```python
from build123d import *

# Parameters (mm, degrees)
SKETCH1_W           = 76.2
SKETCH1_H           = 76.2
BOSS_EXTRUDE1_DEPTH = 3.175
SKETCH2_W           = 50.8
SKETCH2_H           = 50.8
CUT_EXTRUDE1_DEPTH  = 6.35
SKETCH3_R           = 2.159
CUT_EXTRUDE2_DEPTH  = 6.35
SKETCH5_R           = 2.159
CUT_EXTRUDE3_DEPTH  = 6.35
SKETCH6_R           = 2.159
CUT_EXTRUDE4_DEPTH  = 54.975


with BuildPart() as part:
    # Sketch1 → Boss-Extrude1 (new body)
    with BuildSketch(Plane.XY):
        Rectangle(SKETCH1_W, SKETCH1_H)
    extrude(amount=BOSS_EXTRUDE1_DEPTH)

    # Sketch2 → Cut-Extrude1 (cut)
    with BuildSketch(Plane(origin=(0, 0, 0), x_dir=(-1, 0, 0), z_dir=(0, 0, -1))):
        with Locations((12.7, 12.7)):
            Rectangle(SKETCH2_W, SKETCH2_H)
    extrude(amount=-CUT_EXTRUDE1_DEPTH, mode=Mode.SUBTRACT)

    # Sketch3 → Cut-Extrude2 (cut)
    with BuildSketch(Plane(origin=(0, 0, 0), x_dir=(-1, 0, 0), z_dir=(0, 0, -1))):
        with Locations((-25.4, -25.4)):
            Circle(SKETCH3_R)
    extrude(amount=-CUT_EXTRUDE2_DEPTH, mode=Mode.SUBTRACT)

    # Sketch5 → Cut-Extrude3 (cut)
    with BuildSketch(Plane(origin=(0, 0, 0), x_dir=(-1, 0, 0), z_dir=(0, 0, -1))):
        with Locations((24.892, -25.4)):
            Circle(SKETCH5_R)
    extrude(amount=-CUT_EXTRUDE3_DEPTH, mode=Mode.SUBTRACT)

    # Sketch6 → Cut-Extrude4 (cut, through all)
    with BuildSketch(Plane.XY.offset(3.175)):
        with Locations((25.4, 0.508)):
            Circle(SKETCH6_R)
        with Locations((25.4, 24.892)):
            Circle(SKETCH6_R)
    extrude(amount=-CUT_EXTRUDE4_DEPTH, mode=Mode.SUBTRACT)


solid = part.part
```
Geometry: final body of the model. Coordinates: model frame, mm. A direction names the side the tool comes from. Give positions to 0.01 mm unless a question says otherwise; leave off trailing zeros. Loops run counter-clockwise (first coordinate to the right, second up) from the corner with the lowest first, then second, coordinate; pieces in that order, holes last. Notation, with made-up numbers: (-26, 57) - (21, 57) arc R16 ccw to (21, 69) - close; hole circle Ø5 at (24.5, 79). An arc over 180 degrees is marked (long way). Answer as CSV lines item,"result". Start each with the question number.
(1) Section query B-B (x = 25.4). Output: boundary loops of the cut face in (y, z) (3 decimals).
(2) Pin query (flat end, axial travel): P1, Ø2.5, axis at x = 25.4, y = 0.508, coming from the +Z side; P2, Ø7, axis at x = 25.4, y = -25.4, coming from the +Z side (3 decimals); P3, Ø1.6, axis at x = -23.5, z = 2, coming from the +Y side; P4, Ø1, axis at y = 7, z = 1.5, coming from the -X side. Return the tip coordinate at first contact, or that it passes through.
(3) Reachability of faces 1 (the face through (12.7, 12, 2)), 2 (the face through (-38.1, -26, 2)) from +Z, -Z, +X, -X, +Y, -Y: full face, straight path, thin tool, end or side. Return the list, or none.
(4) Ray query, line 1 along Y through (x, z) = (25.4, 1.9); line 2 along X through (y, z) = (-24.5, 2.6); line 3 along X through (y, z) = (14.5, 2.8). Return the intervals inside material, ascending. Write a range as [from, to].
(5) Section query C-C (z = 2.4). Output: boundary loops of the cut face in (x, y).
(6) Section query A-A (y = -25.4). Output: boundary loops of the cut face in (x, z) (3 decimals), and give its area (3 significant figures).
(7) Section query D-D (y = 32). Output: boundary loops of the cut face in (x, z) (3 decimals).
(8) Mould query, pull axis X, two halves, no side actions, for faces 3 (the face through (38.1, -1, 2)), 4 (the face through (-24.61, -23.26, 1.57)), 5 (the face through (25, 38.1, 2)). Classes: +X half, -X half, draft (parallel to the pull), parting line (faces both ways), or undercut.
Worked answers:
1,outline,"(-38.1, 0) - (-27.559, 0) - (-27.559, 3.175) - (-38.1, 3.175) - close; (-23.241, 0) - (-1.651, 0) - (-1.651, 3.175) - (-23.241, 3.175) - close; (2.667, 0) - (22.733, 0) - (22.733, 3.175) - (2.667, 3.175) - close; (27.051, 0) - (38.1, 0) - (38.1, 3.175) - (27.051, 3.175) - close"
2,P1,"passes through"
2,P2,"stops at z = 3.175"
2,P3,"stops at y = -12.7"
2,P4,"stops at x = 12.7"
3,face 1,"+Z, -Z, -X, +Y"
3,face 2,"+Z, -Z, -X, +Y, -Y"
4,line 1,"y = [-38.1, -27.56], [-23.24, -1.65], [2.67, 22.73], [27.05, 38.1]"
4,line 2,"x = [-38.1, -26.85], [-22.93, 23.44], [27.36, 38.1]"
4,line 3,"x = [12.7, 38.1]"
5,outline,"(-38.1, -38.1) - (38.1, -38.1) - (38.1, 38.1) - (12.7, 38.1) - (12.7, -12.7) - (-38.1, -12.7) - close; hole circle Ø4.32 at (-24.89, -25.4); hole circle Ø4.32 at (25.4, -25.4); hole circle Ø4.32 at (25.4, 0.51); hole circle Ø4.32 at (25.4, 24.89)"
6,outline,"(-38.1, 0) - (-27.051, 0) - (-27.051, 3.175) - (-38.1, 3.175) - close; (-22.733, 0) - (23.241, 0) - (23.241, 3.175) - (-22.733, 3.175) - close; (27.559, 0) - (38.1, 0) - (38.1, 3.175) - (27.559, 3.175) - close"
6,area,"215 mm^2"
7,outline,"(12.7, 0) - (38.1, 0) - (38.1, 3.175) - (12.7, 3.175) - close"
8,face 3,"+X half"
8,face 4,"undercut"
8,face 5,"draft"
